Read the model definition and answer for the solid it produces. Units are mm, in the model's axes. A direction names the side the tool comes from. Give positions to 0.01 mm unless a question says otherwise; leave off trailing zeros. Order: outer loops, then holes, each group sorted by start corner. A loop starts at its lowest first (then second) coordinate and runs counter-clockwise, first axis right, second up. Notation, with made-up numbers: (-17, -30) - (32, -30) arc R17 cw to (32, -24) - close; hole circle Ø3 at (-13.75, 44.25). An arc over 180 degrees is marked (long way). Return JSON: item names as keys, results as strings.
Autodesk Inventor part; units mm, degrees
ref_plane "Work Plane1" through (0, 0, 31) normal (0, 0, 1) x (1, 0, 0)
ref_plane "Work Plane2" through (0, 0, 4) normal (0, 0, -1) x (-1, 0, 0)
ref_plane "YZ Plane" through (0, 0, 0) normal (1, 0, 0) x (0, 1, 0)
sketch "Sketch1" plane through (0, 0, 0) normal (0, 0, 1) x (1, 0, 0)
  circle A0 centre (0, 0) radius 3
  circle A1 centre (0, 0) radius 6
  dimension "d0" = 6
  dimension "d1" = 12
extrude "Extrusion1" add sketch "Sketch1" along normal blind 35
ref_plane "Work Plane1" through (0, 0, 31) normal (0, 0, 1) x (1, 0, 0)
ref_plane "Work Plane2" through (0, 0, 4) normal (0, 0, -1) x (-1, 0, 0)
sketch "Sketch2" plane through (0, 0, 31) normal (0, 0, 1) x (1, 0, 0)
  circle A0 centre (0, 0) radius 3
  circle A1 centre (0, 0) radius 6
  circle A2 centre (0, 0) radius 5.5
  circle A3 centre (0, 0) radius 6
  dimension "d6" = 11
extrude "Extrusion2" cut sketch "Sketch2" along normal blind 0.7 contours A1
sketch "Sketch3" plane through (0, 0, 4) normal (0, 0, -1) x (-1, 0, 0)
  circle A0 centre (0, 0) radius 3
  circle A1 centre (0, 0) radius 6
  circle A2 centre (0, 0) radius 5.5
  circle A3 centre (0, 0) radius 6
  dimension "d9" = 11
extrude "Extrusion3" cut sketch "Sketch3" against normal blind 0.7 contours A1
properties part number "LinearBearing"
Q1. Determine the mould class of faces 3 (the cylindrical face through (-3, 0, 17)), 4 (the flat face through (3, -5, 31)), 5 (the cylindrical face through (-6, 0, 2)) for opening direction Y: released by +Y, released by -Y, zero draft, split by the parting line, or undercut.
Values:
{"face 3": "undercut", "face 4": "zero draft", "face 5": "split by the parting line"}
Q2. Consider L1, parallel to Z at x = 4.75, y = -3.25; L2, parallel to Y at x = 0, z = 13; L3, parallel to Y at x = -1.5, z = 8.5. Determine where each line is inside the solid, lowest interval first.
Values:
{"L1": "z = 0 to 4, 4.7 to 31, 31.7 to 35", "L2": "y = -6 to -3, 3 to 6", "L3": "y = -5.81 to -2.6, 2.6 to 5.81"}
Q3. A cutting plane is placed at A-A (y = 0). Write down the section's boundary in (x, z).
Values:
{"outline": "(-6, 0) - (-3, 0) - (-3, 35) - (-6, 35) - (-6, 31.7) - (-5.5, 31.7) - (-5.5, 31) - (-6, 31) - (-6, 4.7) - (-5.5, 4.7) - (-5.5, 4) - (-6, 4) - close; (3, 0) - (6, 0) - (6, 4) - (5.5, 4) - (5.5, 4.7) - (6, 4.7) - (6, 31) - (5.5, 31) - (5.5, 31.7) - (6, 31.7) - (6, 35) - (3, 35) - close"}
Q4. Given pin 1 (3 mm diameter, centred on x = 3.5, z = 31, fed in from +Y); pin 2 (5 mm diameter, centred on y = -3, z = 21.5, fed in from -X); pin 3 (1.5 mm diameter, centred on x = 2.5, z = 22, fed in from -Y), each flat-ended and moving along its own axis, determine where each tip first touches the part or whether it passes through.
Values:
{"pin 1": "stops at y = 5.66", "pin 2": "stops at x = -5.98", "pin 3": "stops at y = -5.74"}
Q5. For faces 1 (the flat face through (3, -5, 31.7)), 2 (the cylindrical face through (-6, 0, 33)), determine the directions among +Z, -Z, +X, -X, +Y, -Y from which every point of the face is accessible in a straight line to the end or side of a thin tool.
Values:
{"face 1": "none", "face 2": "+Z, -Z"}
Q6. A cutting plane is placed at D-D (x = -5). Write down the section's boundary in (y, z), and give its area (3 significant figures).
Values:
{"outline": "(-3.32, 0) - (3.32, 0) - (3.32, 4) - (2.29, 4) - (2.29, 4.7) - (3.32, 4.7) - (3.32, 31) - (2.29, 31) - (2.29, 31.7) - (3.32, 31.7) - (3.32, 35) - (-3.32, 35) - (-3.32, 31.7) - (-2.29, 31.7) - (-2.29, 31) - (-3.32, 31) - (-3.32, 4.7) - (-2.29, 4.7) - (-2.29, 4) - (-3.32, 4) - close", "area": "229 mm²"}
Q7. A cutting plane is placed at C-C (z = 24.5). Write down the section's boundary in (x, y), and give its area (3 significant figures).
Values:
{"outline": "circle Ø12 at (0, 0); hole circle Ø6 at (0, 0)", "area": "84.8 mm²"}
